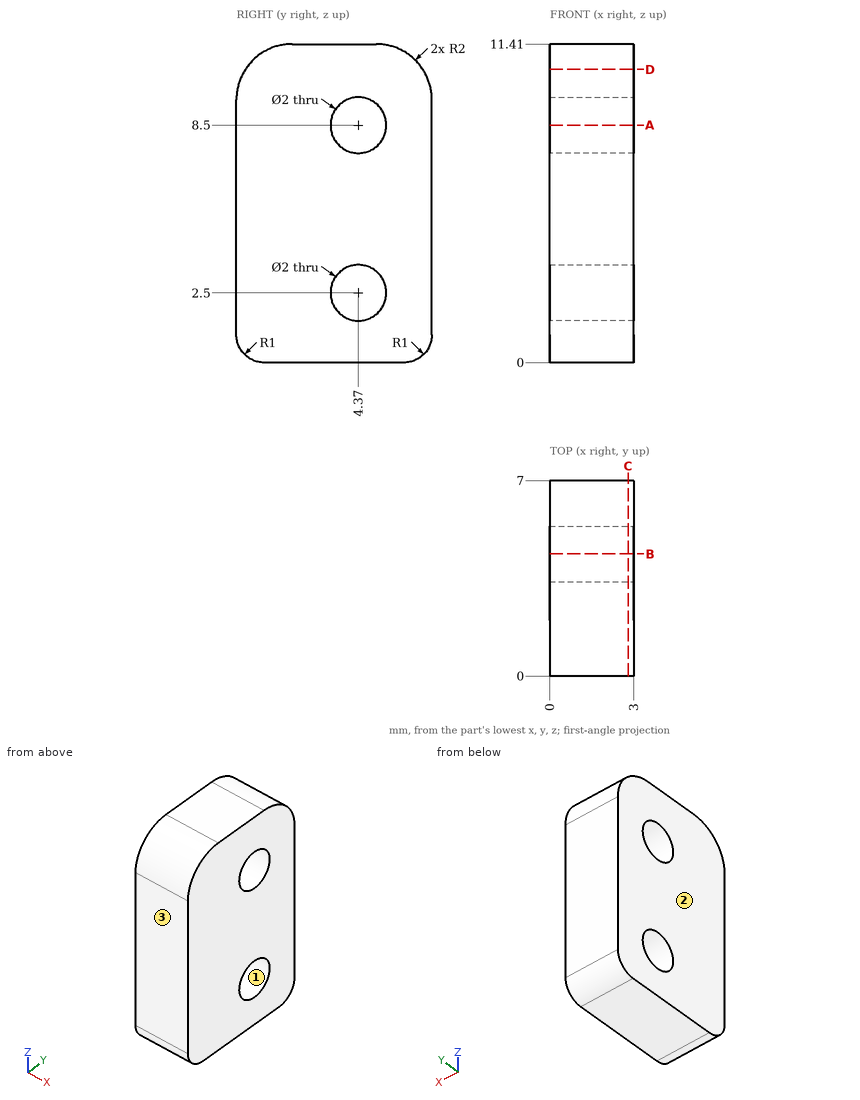
Here's the drawing with two shaded views (mm, measured from the low corner). I have some questions. Round coordinates to 2 decimals unless told otherwise and drop trailing zeros. Loops run counter-clockwise (first coordinate to the right, second up) from the corner with the lowest first, then second, coordinate; pieces in that order, holes last. Notation, with made-up numbers: (62, 62.5) - (66, 62.5) arc R30 ccw to (66, 100.5) - close; hole circle Ø6 at (65, 33). An arc over 180 degrees is marked (long way). Write item = value, one per line.
1) If we mould it in two halves opening along Y, with no side actions, what happens to the marked faces 1, 2 and 3? For each: pulls with the +Y half, pulls with the -Y half, needs draft (parallel to the pull), parting line crosses it, or undercut.
Computed:
face_1 = undercut
face_2 = needs draft
face_3 = pulls with the -Y half
2) Imagine slicing it at C-C (x = 2.8). Please give me the cut outline in (y, z), and give its area (3 significant figures).
Computed:
outline = (0, 1) arc R1 ccw to (1, 0) - (6, 0) arc R1 ccw to (7, 1) - (7, 9.41) arc R2 ccw to (5, 11.41) - (2, 11.41) arc R2 ccw to (0, 9.41) - close; hole circle Ø2 at (4.37, 2.5); hole circle Ø2 at (4.37, 8.5)
area = 71.4 mm2
3) Imagine slicing it at B-B (y = 4.37). Please give me the cut outline in (x, z), and give its area (3 significant figures).
Computed:
outline = (0, 0) - (3, 0) - (3, 1.5) - (0, 1.5) - close; (0, 3.5) - (3, 3.5) - (3, 7.5) - (0, 7.5) - close; (0, 9.5) - (3, 9.5) - (3, 11.41) - (0, 11.41) - close
area = 22.2 mm2
4) Imagine slicing it at A-A (z = 8.5). Please give me the cut outline in (x, y).
Computed:
outline = (0, 0) - (3, 0) - (3, 3.37) - (0, 3.37) - close; (0, 5.37) - (3, 5.37) - (3, 7) - (0, 7) - close
5) Imagine slicing it at D-D (z = 10.5). Please give me the cut outline in (x, y), and give its area (3 significant figures).
Computed:
outline = (0, 0.32) - (3, 0.32) - (3, 6.68) - (0, 6.68) - close
area = 19.1 mm2
6) I need wall thicknesses on line 1 along Y through (x, z) = (1.65, 2.5); line 2 along Z through (x, y) = (0.7, 4.25); line 3 along Z through (x, y) = (2.8, 3.5). Which ranges of each line are inside material? Lowest first, please. Write a range as from..to.
Computed:
line_1 = 0..3.37, 5.37..7
line_2 = 0..1.51, 3.49..7.51, 9.49..11.41
line_3 = 0..2.01, 2.99..8.01, 8.99..11.41
